Here's how the part is built. I have some questions about the finished solid (model axes, mm). A direction names the side the tool comes from. Round coordinates to 2 decimals unless told otherwise and drop trailing zeros. Loops run counter-clockwise (first coordinate to the right, second up) from the corner with the lowest first, then second, coordinate; pieces in that order, holes last. Notation, with made-up numbers: (34.25, 2) -> (56.25, 2) arc R20 ccw to (56.25, 10) -> close; hole circle Ø10 at (-18, 39.25). An arc over 180 degrees is marked (long way). Use CSV: the item, a comma, the result in double quotes. Start each with the question number.
from build123d import *

# Parameters (mm, degrees)
F0_W     = 63.5
F0_H     = 19.05
F0_R     = 6.985
F0_W_2   = 6.35
F0_R_2   = 3.81
F1_DEPTH = 8.255
F2_DEPTH = 25.4
F3_DEPTH = 3.175
F4_R     = 1.8
F5_DEPTH = 6.35
F6_SIZE  = 3.175
F4_R_2   = 3.55
F7_DEPTH = 2.794


with BuildPart() as f1:
    # F0 (on Top) → F1 (new body)
    with BuildSketch(Plane.XY):
        with Locations((3.175, 0)):
            Rectangle(F0_W, F0_H)
        with Locations((24.765, 0)):
            Circle(F0_R, mode=Mode.SUBTRACT)
        with Locations((-31.75, 0)):
            Rectangle(F0_W_2, F0_H)
        with Locations((24.765, 0)):
            Circle(F0_R)
        with Locations((24.765, 0)):
            Circle(F0_R_2, mode=Mode.SUBTRACT)
    extrude(amount=-F1_DEPTH)

    # F0 (on Top) → F2 (join)
    with BuildSketch(Plane.XY):
        with Locations((-31.75, 0)):
            Rectangle(F0_W_2, F0_H)
    extrude(amount=F2_DEPTH)

    # F0 (on Top) → F3 (cut)
    with BuildSketch(Plane.XY):
        with Locations((24.765, 0)):
            Circle(F0_R)
        with Locations((24.765, 0)):
            Circle(F0_R_2, mode=Mode.SUBTRACT)
    extrude(amount=-F3_DEPTH, mode=Mode.SUBTRACT)

    # F4 (on face) → F5 (cut, through all)
    with BuildSketch(Plane.YZ.offset(-28.575)):
        with Locations((0, 6.35)):
            Circle(F4_R)
        with Locations((0, 19.05)):
            Circle(F4_R)
    extrude(amount=-F5_DEPTH, mode=Mode.SUBTRACT)

    # F6
    f6_edges = [f1.edges().sort_by_distance(p)[0] for p in [
        (-28.575, 0, 0),
        (34.925, 9.525, -4.1275),
        (34.925, -9.525, -4.1275),
    ]]
    chamfer(f6_edges, length=F6_SIZE)

    # F4 (on face) → F7 (cut)
    with BuildSketch(Plane.YZ.offset(-28.575)):
        with Locations((0, 6.35)):
            Circle(F4_R_2)
        with Locations((0, 6.35)):
            Circle(F4_R, mode=Mode.SUBTRACT)
        with Locations((0, 19.05)):
            Circle(F4_R_2)
        with Locations((0, 19.05)):
            Circle(F4_R, mode=Mode.SUBTRACT)
    extrude(amount=-F7_DEPTH, mode=Mode.SUBTRACT)


solid = f1.part
Q1. I want a section at B-B, the plane y = 0. Count the separate pieces of the cut face and the enclosed holes in it, then the cut area to 3 significant figures.
Q2. If we mould it in two halves opening along Z, with no side actions, what happens to faces 4 (the cylindrical face through (-33.122, -0.39, 17.293)), 5 (the flat face through (-32, 0, 25.4)), 6 (the flat face through (34.925, 0, -4))? For each: pulls with the +Z half, pulls with the -Z half, needs draft (parallel to the pull), parting line crosses it, or undercut.
Q3. Will these pins go through, and if not, where does the flat tip stop? pin 1 Ø8 at (y, z) = (0, 6.35) entering from +X; pin 2 Ø8 at (y, z) = (-1, 7) entering from +X; pin 3 Ø10 at (x, y) = (-13.5, -3) entering from +Z.
Q4. For faces 1 (the flat face through (-28.575, 0, 14)), 2 (the flat face through (28, -3, -3.175)), 3 (the flat face through (-31.369, -2, 20)), which set-ups out of +Z, -Z, +X, -X, +Y, -Y let a thin tool reach every point of the face, with its end or its side?
Q5. I want a section at A-A, the plane z = 6.35. List the corners of the cut face in (x, y) for me (3 decimals).
Q6. I want a section at D-D, the plane z = -2. List the corners of the cut face in (x, y) for me (3 decimals), then the cut area to 3 significant figures.
Q7. I want a section at C-C, the plane x = 22. List the corners of the cut face in (y, z) for me (3 decimals).
Q8. I need wall thicknesses on line 1 along Z through (x, y) = (-32.5, 0) (3 decimals); line 2 along Z through (x, y) = (-30.8, 0) (3 decimals); line 3 along X through (y, z) = (-4.5, 15.5) (3 decimals). Which ranges of each line are inside material? Lowest first, please.
Values found:
1,separate pieces,"4"
1,enclosed holes,"0"
1,area,"595 mm2"
2,face 4,"undercut"
2,face 5,"pulls with the +Z half"
2,face 6,"needs draft"
3,pin 1,"x = -27.75"
3,pin 2,"x = -28.4"
3,pin 3,"z = 0"
4,face 1,"+Z, +X, +Y, -Y"
4,face 2,"+Z"
4,face 3,"+X"
5,outline,"(-34.925, -9.525) -> (-28.575, -9.525) -> (-28.575, -3.55) -> (-31.369, -3.55) -> (-31.369, -1.8) -> (-34.925, -1.8) -> close; (-34.925, 1.8) -> (-31.369, 1.8) -> (-31.369, 3.55) -> (-28.575, 3.55) -> (-28.575, 9.525) -> (-34.925, 9.525) -> close"
6,outline,"(-34.925, -9.525) -> (31.75, -9.525) -> (34.925, -6.35) -> (34.925, 6.35) -> (31.75, 9.525) -> (-34.925, 9.525) -> close; hole circle Ø13.97 at (24.765, 0)"
6,area,"1,170 mm2"
7,outline,"(-9.525, -8.255) -> (-2.621, -8.255) -> (-2.621, -3.175) -> (-6.414, -3.175) -> (-6.414, 0) -> (-9.525, 0) -> close; (2.621, -8.255) -> (9.525, -8.255) -> (9.525, 0) -> (6.414, 0) -> (6.414, -3.175) -> (2.621, -3.175) -> close"
8,line 1,"-8.255 to 4.55, 8.15 to 17.25, 20.85 to 25.4"
8,line 2,"-8.255 to 2.8, 9.9 to 15.5, 22.6 to 25.4"
8,line 3,"-34.925 to -28.575"
